from build123d import *

# Parameters (mm, degrees)
CROQUIS1_R              = 5
SALIENTE_EXTRUIR1_DEPTH = 10


with BuildPart() as part:
    # Croquis1 → Saliente-Extruir1 (new body)
    with BuildSketch(Plane.XY):
        with BuildLine():
            ThreePointArc((8.081598806, 65.88963163), (0, 70), (-8.081598806, 65.88963163))
            ThreePointArc((-8.081598806, 65.88963163), (-27.803831164, 48.157648221), (-53.021295435, 39.943685684))
            ThreePointArc((-53.021295435, 39.943685684), (-60.621778265, 35), (-61.102894241, 25.945945946))
            ThreePointArc((-61.102894241, 25.945945946), (-55.607662328, 0), (-61.102894241, -25.945945946))
            ThreePointArc((-61.102894241, -25.945945946), (-60.621778265, -35), (-53.021295435, -39.943685684))
            ThreePointArc((-53.021295435, -39.943685684), (-27.803831164, -48.157648221), (-8.081598806, -65.88963163))
            ThreePointArc((-8.081598806, -65.88963163), (0, -70), (8.081598806, -65.88963163))
            ThreePointArc((8.081598806, -65.88963163), (27.803831164, -48.157648221), (53.021295435, -39.943685684))
            ThreePointArc((53.021295435, -39.943685684), (60.621778265, -35), (61.102894241, -25.945945946))
            ThreePointArc((61.102894241, -25.945945946), (55.607662328, 0), (61.102894241, 25.945945946))
            ThreePointArc((61.102894241, 25.945945946), (60.621778265, 35), (53.021295435, 39.943685684))
            ThreePointArc((53.021295435, 39.943685684), (27.803831164, 48.157648221), (8.081598806, 65.88963163))
        make_face()
        with Locations((0, 60)):
            Circle(CROQUIS1_R, mode=Mode.SUBTRACT)
        with Locations((51.961524227, 30)):
            Circle(CROQUIS1_R, mode=Mode.SUBTRACT)
        with Locations((51.961524227, -30)):
            Circle(CROQUIS1_R, mode=Mode.SUBTRACT)
        with Locations((0, -60)):
            Circle(CROQUIS1_R, mode=Mode.SUBTRACT)
        with Locations((-51.961524227, -30)):
            Circle(CROQUIS1_R, mode=Mode.SUBTRACT)
        with Locations((-51.961524227, 30)):
            Circle(CROQUIS1_R, mode=Mode.SUBTRACT)
        with BuildLine():
            Line((27.966013781, 15.553201382), (21.14530514, 13.337018802))
            ThreePointArc((21.14530514, 13.337018802), (14.694631307, 20.225424859), (6.15, 24.231745707))
            Line((6.15, 24.231745707), (6.15, 31.403463185))
            ThreePointArc((6.15, 31.403463185), (0, 32), (-6.15, 31.403463185))
            Line((-6.15, 31.403463185), (-6.15, 24.231745707))
            ThreePointArc((-6.15, 24.231745707), (-14.694631307, 20.225424859), (-21.14530514, 13.337018802))
            Line((-21.14530514, 13.337018802), (-27.966013781, 15.553201382))
            ThreePointArc((-27.966013781, 15.553201382), (-30.433808521, 9.88854382), (-31.766922812, 3.855206231))
            Line((-31.766922812, 3.855206231), (-24.946214171, 1.639023652))
            ThreePointArc((-24.946214171, 1.639023652), (-23.776412907, -7.725424859), (-19.218517279, -15.989014779))
            Line((-19.218517279, -15.989014779), (-23.433947046, -21.791056097))
            ThreePointArc((-23.433947046, -21.791056097), (-18.809128073, -25.88854382), (-13.483038016, -29.0208147))
            Line((-13.483038016, -29.0208147), (-9.267608248, -23.218773382))
            ThreePointArc((-9.267608248, -23.218773382), (0, -25), (9.267608248, -23.218773382))
            Line((9.267608248, -23.218773382), (13.483038016, -29.0208147))
            ThreePointArc((13.483038016, -29.0208147), (18.809128073, -25.88854382), (23.433947046, -21.791056097))
            Line((23.433947046, -21.791056097), (19.218517279, -15.989014779))
            ThreePointArc((19.218517279, -15.989014779), (23.776412907, -7.725424859), (24.946214171, 1.639023652))
            Line((24.946214171, 1.639023652), (31.766922812, 3.855206231))
            ThreePointArc((31.766922812, 3.855206231), (30.433808521, 9.88854382), (27.966013781, 15.553201382))
        make_face(mode=Mode.SUBTRACT)
    extrude(amount=SALIENTE_EXTRUIR1_DEPTH)


solid = part.part
The listing builds one solid part. Answer for the finished solid, in the listing's coordinates (mm). A direction names the side the tool comes from. Give positions to 0.01 mm unless a question says otherwise; leave off trailing zeros. Write each loop counter-clockwise with the first axis right and the second up, starting at its lowest first coordinate (ties: lowest second). Pieces come first, ordered by that corner, then holes.
1) Section A-A (x = 0) is taken. Write down the section's boundary in (y, z), and give its area (3 significant figures).
2) For a pull along X with two mould halves and no side action, classify faces 3 (the face through (24.6, 14.46, 4.93)), 4 (the face through (60.555, -35.114, 4.93)), 5 (the face through (0, -70, 5)), 6 (the face through (27, 1, 0)) as pulls with the +X half, pulls with the -X half, needs draft (parallel to the pull), parting line crosses it, or undercut.
3) A tool of negligible diameter and unlimited length cuts with its end or side. For faces 1 (the face through (0, 70, 5)), 2 (the face through (-15, 20, 5)), from which of +Z, -Z, +X, -X, +Y, -Y can it reach the whole face along a straight path? Write none if from no direction.
4) Section B-B (y = 60) is taken. Write down the section's boundary in (x, z), and give its area (3 significant figures).
5) Section C-C (z = 5.75) is taken. Count the separate pieces of the cut face and the enclosed holes in it, and give its area (3 significant figures).
6) Section D-D (x = 33.5) is taken. Write down the section's boundary in (y, z), and give its area (3 significant figures).
7) Given P1, Ø9, axis at x = -51.96, y = 30, coming from the -Z side; P2, Ø3.5, axis at y = 27.5, z = 4.5, coming from the -X side; P3, Ø6, axis at y = -22.5, z = 3, coming from the -X side; P4, Ø3, axis at y = -18.5, z = 2.5, coming from the +X side, each flat-ended and moving along its own axis, determine where each tip first touches the part or whether it passes through.
8) Find the intervals of material crossed by L1, parallel to X at y = -2, z = 7; L2, parallel to Y at x = 51, z = 5; L3, parallel to X at y = -28.5, z = 7.5, in increasing order.
Response:
1. outline: (-70, 0) - (-65, 0) - (-65, 10) - (-70, 10) - close; (-55, 0) - (-25, 0) - (-25, 10) - (-55, 10) - close; (32, 0) - (55, 0) - (55, 10) - (32, 10) - close; (65, 0) - (70, 0) - (70, 10) - (65, 10) - close
1. area: 630 mm2
2. face 3: undercut
2. face 4: pulls with the +X half
2. face 5: parting line crosses it
2. face 6: needs draft
3. face 1: +Z, -Z, +Y
3. face 2: +Z, -Z
4. outline: (-12.94, 0) - (-5, 0) - (-5, 10) - (-12.94, 10) - close; (5, 0) - (12.94, 0) - (12.94, 10) - (5, 10) - close
4. area: 159 mm2
5. separate pieces: 1
5. enclosed holes: 7
5. area: 8,970 mm2
6. outline: (-45.24, 0) - (45.24, 0) - (45.24, 10) - (-45.24, 10) - close
6. area: 905 mm2
7. P1: passes through
7. P2: stops at x = -61.93
7. P3: stops at x = -60.91
7. P4: stops at x = 58.81
8. L1: x = -55.64 to -24.92, 24.92 to 55.64
8. L2: y = -40.19 to -34.91, -25.09 to 25.09, 34.91 to 40.19
8. L3: x = -61.85 to -56.73, -47.19 to -14.55, -13.1 to 13.1, 14.55 to 47.19, 56.73 to 61.85
